Autodesk Inventor part; units mm, degrees
ref_plane "YZ Plane" through (0, 0, 0) normal (1, 0, 0) x (0, 1, 0)
ref_plane "XZ Plane" through (0, 0, 0) normal (0, 1, 0) x (-1, 0, 0)
ref_plane "XY Plane" through (0, 0, 0) normal (0, 0, 1) x (1, 0, 0)
sketch "Sketch1" plane through (0, 0, 0) normal (0, 1, 0) x (-1, 0, 0)
  line L0 (-89, 127) -> (89, 127)
  line L1 (89, 127) -> (89, -127)
  line L2 (89, -127) -> (-89, -127)
  line L3 (-89, -127) -> (-89, 127)
  line L4 (-89, 127) -> (89, -127) construction
  line L5 (89, 127) -> (-89, -127) construction
  line L6 (90, 128) -> (-90, 128)
  line L7 (-90, 128) -> (-90, -128)
  line L8 (-90, -128) -> (90, -128)
  line L9 (90, -128) -> (90, 128)
  point P0 (0, 0)
  dimension "d0" = 178
  dimension "d1" = 254
  dimension "d2" = 1
extrude "Extrusion1" add sketch "Sketch1" along normal blind 101.6
sketch "Sketch3" plane through (0, 0, 0) normal (0, -1, 0) x (1, 0, 0)
  line L0 (90, 128) -> (90, -128)
  line L1 (90, -128) -> (-90, -128)
  line L2 (90, 128) -> (90, -128)
  line L3 (90, -128) -> (115, -128)
  line L4 (115, -128) -> (115, 128)
  line L5 (115, 128) -> (90, 128)
  line L6 (90, -128) -> (-90, -128)
  line L7 (-90, -128) -> (-90, -153)
  line L8 (-90, -153) -> (90, -153)
  line L9 (90, -153) -> (90, -128)
  line L10 (-90, 128) -> (90, 128)
  line L11 (-90, -128) -> (-90, 128)
  line L12 (-90, 128) -> (-115, 128)
  line L13 (-115, 128) -> (-115, -128)
  line L14 (-115, -128) -> (-90, -128)
  line L15 (-90, 128) -> (90, 128)
  line L16 (90, 128) -> (90, 153)
  line L17 (90, 153) -> (-90, 153)
  line L18 (-90, 153) -> (-90, 128)
  point P0 (0, 0)
  dimension "d11" = 25
  dimension "d12" = 25
  dimension "d13" = 25
  dimension "d14" = 25
extrude "Extrusion3" add sketch "Sketch3" against normal blind 0.8 contours L5 L4 L3 L0 | L10 L18 L17 L16 | L9 L8 L7 L1 | L11 L14 L13 L12
sketch "Sketch4" plane through (0, 0.8, 0) normal (0, 1, 0) x (1, 0, 0)
  line L0 (101.5, 139.5) -> (-101.5, 139.5) construction
  line L1 (-101.5, 139.5) -> (-101.5, -139.5) construction
  line L2 (-101.5, -139.5) -> (101.5, -139.5) construction
  line L3 (101.5, -139.5) -> (101.5, 139.5) construction
  line L4 (101.5, 139.5) -> (-101.5, -139.5) construction
  line L5 (-101.5, 139.5) -> (101.5, -139.5) construction
  line L6 (0, 0) -> (0, -60) construction
  line L7 (0, 0) -> (60, 0) construction
  point P0 (-101.5, 0)
  point P1 (101.5, 0)
  point P2 (101.5, 104.625)
  point P3 (101.5, 69.75)
  point P4 (101.5, 34.875)
  point P5 (101.5, 0)
  point P6 (101.5, -34.875)
  point P7 (101.5, -69.75)
  point P8 (101.5, -104.625)
  point P9 (67.6667, 139.5)
  point P10 (33.8333, 139.5)
  point P11 (0, 139.5)
  point P12 (-33.8333, 139.5)
  point P13 (-67.6667, 139.5)
  point P14 (-101.5, 139.5)
  point P15 (67.6667, -139.5)
  point P16 (33.8333, -139.5)
  point P17 (0, -139.5)
  point P18 (-33.8333, -139.5)
  point P19 (-67.6667, -139.5)
  point P20 (-101.5, -139.5)
  point P21 (-101.5, 104.625)
  point P22 (-101.5, 69.75)
  point P23 (-101.5, 34.875)
  point P24 (-101.5, 0)
  point P25 (-101.5, -34.875)
  point P26 (-101.5, -69.75)
  point P27 (-101.5, -104.625)
  dimension "d18" = 203
  dimension "d19" = 279
  dimension "d21" = 60
  dimension "d22" = 90
  dimension "d63" = 34.875
  dimension "d70" = 33.8333
  dimension "d77" = 33.8333
  dimension "d84" = 34.875
hole "Hole1" at (101.5, 0.8, -139.5) at (101.5, 0.8, -104.625) at (101.5, 0.8, -34.875) at (101.5, 0.8, 34.875) at (101.5, 0.8, 104.625) at (101.5, 0.8, 139.5) at (67.6667, 0.8, -139.5) at (0, 0.8, -139.5) at (-67.6667, 0.8, -139.5) at (-101.5, 0.8, -139.5) at (67.6667, 0.8, 139.5) at (0, 0.8, 139.5) at (-67.6667, 0.8, 139.5) at (-101.5, 0.8, 139.5) at (-101.5, 0.8, -104.625) at (-101.5, 0.8, -34.875) at (-101.5, 0.8, 34.875) at (-101.5, 0.8, 104.625) direction (0, -1, 0) diameter 6 end through all
sketch "Sketch9" plane through (90, 0.8, 128) normal (1, 0, 0) x (0, 0, -1)
  line L0 (0, 100.8) -> (19.3185, 105.9764)
  line L1 (0, 100.8) -> (20, 100.8) construction
  line L2 (19.3721, 105.7764) -> (0.8, 100.8)
  line L3 (19.3185, 105.9764) -> (19.3721, 105.7764)
  line L4 (256, 0) -> (256, 100.8)
  line L5 (256, 100.8) -> (236.6815, 105.9764)
  line L6 (256, 100.8) -> (276, 100.8) construction
  line L7 (0, 100.8) -> (256, 100.8)
  line L8 (229, 100.8) -> (256, 100.8)
  line L9 (256, 100.8) -> (0, 100.8)
  line L10 (0, 100.8) -> (0.8, 100.8)
  line L11 (236.4744, 105.2036) -> (252.909, 100.8)
  line L12 (236.6815, 105.9764) -> (236.4744, 105.2036)
  point P0 (128, -0.8)
  dimension "d51" = 20
  dimension "d52" = 15
  dimension "d53" = 20
  dimension "d54" = 165
  dimension "d89" = 0.8
extrude "Extrusion10" add sketch "Sketch9" against normal up to surface (180 mm away)
properties part number "chimneyHousing"
Geometry: final body of the model. Coordinates: model frame, mm. A direction names the side the tool comes from. Round coordinates to 2 decimals unless told otherwise and drop trailing zeros. Order: outer loops, then holes, each group sorted by start corner. A loop starts at its lowest first (then second) coordinate and runs counter-clockwise, first axis right, second up. Notation, with made-up numbers: (52.5, -9.75) -> (99.5, -9.75) arc R29 ccw to (99.5, 27.25) -> close; hole circle Ø6 at (74.5, -11.5). An arc over 180 degrees is marked (long way). Use CSV: the item, a comma, the result in double quotes. Start each with the question number.
1) Section B-B (z = 14). Return the cut outline in (x, y).
2) Set-up query: faces 5 (the face through (-1, 0.8, -143)), 6 (the face through (90, 53, 2)), 7 (the face through (-1, 50, -127)). Return all of +Z, -Z, +X, -X, +Y, -Y with unobstructed straight access to the full face (end or side cutting, diameter ignored); none if empty.
3) Section A-A (x = -51.5). Return the cut outline in (y, z), and give its area (3 significant figures).
4) Draft query along Z for faces 1 (the face through (-1, 50, 128)), 2 (the face through (-94, 0, 1)), 3 (the face through (89, 50, -2)), 4 (the face through (1, 50, 127)). Return one class per face: +Z half, -Z half, draft (parallel to the pull), parting line (faces both ways), or undercut.
5) Material intervals for line 1 along X through (y, z) = (0.3, 139.5); line 2 along X through (y, z) = (79.5, 14); line 3 along Z through (x, y) = (-19, 100), sorted ascending. Write a range as from..to.
6) Section C-C (y = 89.5). Return the cut outline in (x, z), and give its area (3 significant figures).
7) First-contact query: pin 1 Ø1 at (x, z) = (-9.5, 111.5) entering from -Y; pin 2 Ø1.5 at (x, y) = (-11, 55.5) entering from +Z; pin 3 Ø2 at (x, z) = (-79, 108.5) entering from -Y. Flat tips, straight axial feed; report the tip coordinate or a pass-through.
Returned:
1,outline,"(-115, 0) -> (-89, 0) -> (-89, 101.6) -> (-90, 101.6) -> (-90, 0.8) -> (-115, 0.8) -> close; (89, 0) -> (115, 0) -> (115, 0.8) -> (90, 0.8) -> (90, 101.6) -> (89, 101.6) -> close"
2,face 5,"-Z, +X, -X, +Y"
2,face 6,"+Z, -Z, +X, +Y"
2,face 7,"-Y"
3,outline,"(0, -153) -> (0.8, -153) -> (0.8, -128) -> (101.6, -128) -> (106.78, -108.68) -> (106, -108.47) -> (101.6, -124.91) -> (101.6, -127) -> (0, -127) -> close; (0, 127) -> (101.6, 127) -> (101.6, 127.2) -> (106.58, 108.63) -> (106.78, 108.68) -> (101.6, 128) -> (0.8, 128) -> (0.8, 153) -> (0, 153) -> close"
3,area,"262 mm²"
4,face 1,"+Z half"
4,face 2,"draft"
4,face 3,"undercut"
4,face 4,"undercut"
5,line 1,"x = -90..-70.67, -64.67..-3, 3..64.67, 70.67..90"
5,line 2,"x = -90..-89, 89..90"
5,line 3,"z = -128..-127, 127..128"
6,outline,"(-90, -128) -> (90, -128) -> (90, 128) -> (-90, 128) -> close; hole (-89, -127) -> (89, -127) -> (89, 127) -> (-89, 127) -> close"
6,area,"868 mm²"
7,pin 1,"stops at y = 105.67"
7,pin 2,"stops at z = 128"
7,pin 3,"stops at y = 106.34"
